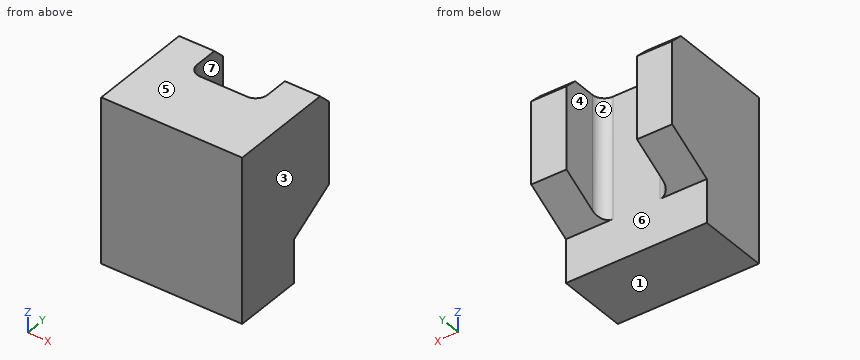
Autodesk Inventor part; units mm, degrees
ref_plane "YZ Plane" through (0, 0, 0) normal (1, 0, 0) x (0, 1, 0)
ref_plane "XZ Plane" through (0, 0, 0) normal (0, 1, 0) x (-1, 0, 0)
ref_plane "XY Plane" through (0, 0, 0) normal (0, 0, 1) x (1, 0, 0)
sketch "Esboço1" plane through (0, 0, 0) normal (0, 1, 0) x (-1, 0, 0)
  line L0 (30, -35) -> (-30, -35)
  line L1 (-30, -35) -> (-30, 35)
  line L2 (-30, 35) -> (30, 35)
  line L3 (30, 35) -> (30, -35)
  line L4 (30, -35) -> (-30, 35) construction
  line L5 (-30, -35) -> (30, 35) construction
  point P0 (0, 0)
  dimension "d0" = 60
  dimension "d1" = 70
extrude "Extrusão1" add sketch "Esboço1" along normal blind 50
sketch "Esboço3" plane through (30, 0, 35) normal (1, 0, 0) x (0, 0, -1)
  line L0 (0, 50) -> (70, 50)
  line L1 (40, 50) -> (51.547, 30)
  line L2 (51.547, 30) -> (70, 30)
  line L3 (40, 50) -> (70, 50)
  line L4 (70, 0) -> (70, 50)
  line L5 (70, 30) -> (70, 50)
  point P0 (35, 0)
  dimension "d6" = 20
  dimension "d7" = 30
  dimension "d8" = 60
extrude "Extrusão2" cut sketch "Esboço3" against normal through all
sketch "Esboço4" plane through (-30, 0, 35) normal (0, 0, 1) x (1, 0, 0)
  line L0 (15, 50) -> (45, 50)
  line L1 (45, 50) -> (45, 30)
  line L2 (45, 30) -> (15, 30)
  line L3 (15, 30) -> (15, 50)
  line L4 (0, 50) -> (60, 50)
  point P0 (30, 0)
  point P1 (30, 50)
  dimension "d11" = 30
  dimension "d12" = 20
extrude "Extrusão3" cut sketch "Esboço4" against normal through all
fillet "Arredondamento1" radius 5 2 edges at (-15, 30, 9.2265) (15, 30, 9.2265)
chamfer "Chanfro1" distance 5 angle 45 2 edges at (-22.5, 50, 35) (22.5, 50, 35)
properties part number "3D Model"
Verification items for the finished model (mm, model axes). Face numbers are marked on the shaded views. A direction names the side the tool comes from. Coordinates: 2 decimals unless noted, no trailing zeros. Loops run counter-clockwise (first coordinate to the right, second up) from the corner with the lowest first, then second, coordinate; pieces in that order, holes last. Notation, with made-up numbers: (-1.75, 6) -> (4.25, 6) arc R24 cw to (4.25, 20) -> close; hole circle Ø1 at (-22, 51). An arc over 180 degrees is marked (long way). Answer in a Markdown table with one row per item. Add a question column.
1. Access from +Z, -Z, +X, -X, +Y, -Y to the whole of each face (thin tool, end or side, straight path). Record for the marked faces 5, 6 and 7.
2. Draft check along X on the marked faces 1, 2, 3 and 4. Enter one of: +X half, -X half, draft (parallel to the pull), parting line (faces both ways), or undercut.
3. Material ranges on probe 1 along X at (y, z) = (38, 0); probe 2 along Y at (x, z) = (4.5, 7); probe 3 along Y at (x, z) = (-17.5, -8.5), recorded low to high. Write a range as [from, to].
4. Depth check by flat-ended pin: P1, Ø1, axis at x = 12.5, z = -20, coming from the +Y side. Enter the tip coordinate at first touch or a pass-through.
5. Section check A-A, the plane z = -4. Enter the section's corners in (x, y), then the cut area to 3 significant figures.
6. Section check B-B, the plane y = 37. Enter the section's corners in (x, z), then the cut area to 3 significant figures.
7. Section check C-C, the plane x = 24. Enter the section's corners in (y, z).
8. Section check D-D, the plane x = 2.5. Enter the section's corners in (y, z), then the cut area to 3 significant figures.
Derived:
| question | item | result |
|---|---|---|
| 1 | face 5 | +Z, +X, -X, +Y, -Y |
| 1 | face 6 | -Z, +Y |
| 1 | face 7 | +Z, -Z, +Y |
| 2 | face 1 | draft |
| 2 | face 2 | undercut |
| 2 | face 3 | +X half |
| 2 | face 4 | undercut |
| 3 | probe 1 | x = [-30, -15], [15, 30] |
| 3 | probe 2 | y = [0, 30] |
| 3 | probe 3 | y = [0, 43.94] |
| 4 | P1 | stops at y = 30 |
| 5 | outline | (-30, 0) -> (30, 0) -> (30, 50) -> (15, 50) -> (15, 35) arc R5 cw to (10, 30) -> (-10, 30) arc R5 cw to (-15, 35) -> (-15, 50) -> (-30, 50) -> close |
| 5 | area | 2,410 mm² |
| 6 | outline | (-30, -12.51) -> (-15, -12.51) -> (-15, 35) -> (-30, 35) -> close; (15, -12.51) -> (30, -12.51) -> (30, 35) -> (15, 35) -> close |
| 6 | area | 1,430 mm² |
| 7 | outline | (0, -35) -> (30, -35) -> (30, -16.55) -> (50, -5) -> (50, 30) -> (45, 35) -> (0, 35) -> close |
| 8 | outline | (0, -35) -> (30, -35) -> (30, 35) -> (0, 35) -> close |
| 8 | area | 2,100 mm² |
